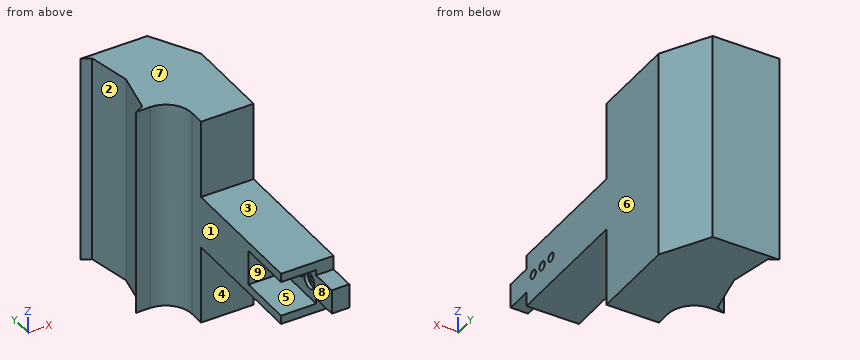
Autodesk Inventor part; units mm, degrees
ref_plane "Work Plane1" through (0, 0, -15) normal (0, 0, 1) x (1, 0, 0)
ref_plane "YZ Plane" through (0, 0, 0) normal (1, 0, 0) x (0, 1, 0)
ref_plane "XZ Plane" through (0, 0, 0) normal (0, 1, 0) x (-1, 0, 0)
sketch "Sketch1" plane through (0, 0, 0) normal (0, 0, 1) x (1, 0, 0)
  line L0 (0, 0) -> (25, 0)
  line L1 (25, 0) -> (25, 40)
  line L2 (25, 40) -> (0, 40)
  line L3 (0, 40) -> (0, 0)
  dimension "d1" = 25
  dimension "d2" = 40
  dimension "d3" = 25
extrude "Extrusion1" add sketch "Sketch1" against normal blind 30
sketch "Sketch2" plane through (25, 0, 0) normal (1, 0, 0) x (0, 0, -1)
  line L0 (0, 0) -> (30, 0)
  circle A0 centre (15, 6.56) radius 2.46
extrude "Extrusion2" cut sketch "Sketch2" against normal blind 30
sketch "Sketch3" plane through (0, 0, 0) normal (-1, 0, 0) x (0, 0, 1)
  line L0 (0, 0) -> (-30, 0)
  line L1 (-25.05, 0) -> (-4.95, 0)
  line L2 (-4.95, 0) -> (-4.95, 33.12)
  line L3 (-4.95, 33.12) -> (-25.05, 33.12)
  line L4 (-25.05, 33.12) -> (-25.05, 0)
  dimension "d11" = 20.1
extrude "Extrusion3" cut sketch "Sketch3" against normal blind 20
sketch "Sketch4" plane through (0, 0, 0) normal (0, -1, 0) x (1, 0, 0)
  line L0 (20, -4.95) -> (20, -25.05)
  line L1 (20, -15) -> (25, -15)
  line L2 (25, 0) -> (25, -30)
  line L3 (20, -8.025) -> (25, -8.025)
  line L4 (25, -8.025) -> (25, -21.975)
  line L5 (25, -21.975) -> (20, -21.975)
  line L6 (20, -21.975) -> (20, -8.025)
  line L7 (20, -8.025) -> (25, -21.975) construction
  line L8 (25, -8.025) -> (20, -21.975) construction
  line L9 (25, -12.54) -> (25, -17.46)
  point P0 (0, 0)
  point P1 (22.5, -15)
  dimension "d14" = 13.95
extrude "Extrusion4" add sketch "Sketch4" along normal blind 15
sketch "Sketch5" plane through (20, 0, 0) normal (-1, 0, 0) x (0, 0, 1)
  circle A0 centre (-15, 6.56) radius 2.46
  circle A1 centre (-15, 6.56) radius 4.7025
  circle A2 centre (-15, 6.56) radius 2.46
  circle A3 centre (-15, 6.56) radius 2.46
  point P0 (0, 0)
  dimension "d17" = 9.405
extrude "Extrusion5" cut sketch "Sketch5" against normal blind 2.1
sketch "Sketch6" plane through (25, 0, 0) normal (1, 0, 0) x (0, 0, -1)
  circle A0 centre (15, 6.56) radius 4.7025
  line L0 (15, 6.56) -> (15, 23.56)
  circle A1 centre (15, 23.56) radius 2.46
  point P0 (0, 0)
  dimension "d20" = 17
  dimension "d21" = 4.92
extrude "Extrusion6" cut sketch "Sketch6" against normal blind 10 contours A1
sketch "Sketch7" plane through (20, 0, 0) normal (-1, 0, 0) x (0, 0, 1)
  circle A0 centre (-15, 23.56) radius 2.46
  circle A1 centre (-15, 23.56) radius 4.7025
  point P0 (0, 0)
  dimension "d24" = 9.405
extrude "Extrusion7" cut sketch "Sketch7" against normal blind 2.1
sketch "Sketch9" plane through (25, 0, 0) normal (1, 0, 0) x (0, 0, -1)
  circle A0 centre (15, 6.56) radius 2.46
  circle A1 centre (15, 6.56) radius 2.46
  circle A2 centre (15, 23.56) radius 2.46
  circle A3 centre (15, 23.56) radius 2.46
  line L0 (30, 40) -> (30, 0)
  line L1 (30, 0) -> (30, 40)
  line L2 (30, 40) -> (0, 40)
  line L3 (0, 40) -> (0, 0)
  line L4 (0, 0) -> (8.025, 0)
  line L5 (21.975, 0) -> (21.975, -15)
  line L6 (21.975, -15) -> (8.025, -15)
  line L7 (8.025, -15) -> (8.025, 0)
  line L8 (0, 0) -> (8.025, 0)
  line L9 (21.975, 0) -> (30, 0)
extrude "Extrusion8" add sketch "Sketch9" along normal blind 5
sketch "Sketch10" plane through (0, 40, 0) normal (0, 1, 0) x (1, 0, 0)
  line L0 (0, 30) -> (30, 30)
  line L1 (30, 0) -> (0, 0)
  line L2 (0, 30) -> (30, 30)
  line L3 (30, 30) -> (30, 0)
  line L4 (30, 0) -> (0, 0)
  line L5 (0, 0) -> (0, 30)
extrude "Extrusion9" add sketch "Sketch10" along normal blind 30
sketch "Sketch12" plane through (30, 0, 0) normal (1, 0, 0) x (0, 0, -1)
  circle A0 centre (15, 6.56) radius 2.46
  line L0 (15, 6.56) -> (15, 15.06)
  circle A1 centre (15, 15.06) radius 2.525
  point P0 (0, 0)
  dimension "d31" = 8.5
  dimension "d33" = 5.05
extrude "Extrusion10" cut sketch "Sketch12" against normal blind 30 contours A1
sketch "Sketch14" plane through (0, 0, 0) normal (0, 0, 1) x (1, 0, 0)
  line L0 (30, 70) -> (0, 70)
  line L1 (0, 70) -> (0, 85)
  line L2 (-15, 100) -> (-23, 100)
  line L3 (30, 0) -> (30, 70)
  line L4 (30, 122.5) -> (30, 70)
  arc A0 (0, 85) -> (-15, 100) centre (-15, 85) ccw
  line L5 (30, 105) -> (30, 100)
  line L6 (-23, 153) -> (15, 153)
  line L7 (-18, 150.5) -> (-23, 153)
  line L8 (-18, 102.5) -> (-23, 100)
  line L9 (-18, 102.5) -> (-13, 126.5)
  line L10 (-13, 126.5) -> (-18, 150.5)
  line L11 (30, 126.5) -> (15, 153)
  line L12 (30, 122.5) -> (30, 126.5)
  point P0 (0, 0)
  point P1 (0, 100)
  dimension "d47" = 30
  dimension "d54" = 15
extrude "Extrusion12" add sketch "Sketch14" against normal blind 30
sketch "Sketch15" plane through (0, 0, -25.05) normal (-1, 0, 0) x (0, 0, 1)
  line L0 (0, 33.12) -> (20.1, 33.12)
  line L1 (20.1, 33.12) -> (20.1, 0)
  line L2 (0, 33.12) -> (20.1, 33.12)
  line L3 (20.1, 33.12) -> (20.1, 31.1)
  line L4 (20.1, 31.1) -> (0, 31.1)
  line L5 (0, 31.1) -> (0, 33.12)
  point P0 (25.05, 0)
  dimension "d57" = 2.02
extrude "Extrusion13" add sketch "Sketch15" against normal blind 20
sketch "Sketch25" plane through (0, 0, 0) normal (0, 0, 1) x (1, 0, 0)
  line L0 (-15, 100) -> (-23, 100)
  line L1 (-15, 100) -> (-23, 100)
  line L2 (-23, 100) -> (-18, 102.5)
  line L3 (-23, 100) -> (-18, 102.5)
  line L4 (-18, 102.5) -> (-13, 126.5)
  line L5 (-18, 102.5) -> (-13, 126.5)
  line L6 (-13, 126.5) -> (-18, 150.5)
  line L7 (-13, 126.5) -> (-18, 150.5)
  line L8 (-18, 150.5) -> (-23, 153)
  line L9 (-18, 150.5) -> (-23, 153)
  line L10 (-23, 153) -> (15, 153)
  line L11 (-23, 153) -> (15, 153)
  line L12 (15, 153) -> (30, 126.5)
  line L13 (15, 153) -> (30, 126.5)
  line L14 (30, 126.5) -> (30, 76.5)
  line L15 (30, 0) -> (30, 126.5)
  line L16 (30, 76.5) -> (0, 76.5)
  arc A0 (0, 85) -> (-15, 100) centre (-15, 85) ccw
  line L17 (0, 76.5) -> (0, 85)
  line L18 (0, 85) -> (0, 0)
  arc A1 (0, 85) -> (-15, 100) centre (-15, 85) ccw
  dimension "d90" = 50
extrude "Extrusion14" add sketch "Sketch25" along normal blind 45
ref_plane "Work Plane1" through (0, 0, -15) normal (0, 0, 1) x (1, 0, 0)
mirror "Mirror1" about plane through (0, 0, -15) normal (0, 0, 1) of "Extrusion14"
properties part number "rec_a_48mm_x_120mm"
Read the model definition and answer for the solid it produces. Units are mm, in the model's axes. Face numbers are marked on the shaded views. A direction names the side the tool comes from. Give positions to 0.01 mm unless a question says otherwise; leave off trailing zeros. Loops run counter-clockwise (first coordinate to the right, second up) from the corner with the lowest first, then second, coordinate; pieces in that order, holes last.
Item 1: Find the intervals of material crossed by line 1 along Z through (x, y) = (21, 23); line 2 along Z through (x, y) = (24.25, 23.56); line 3 along Y through (x, z) = (25.25, -15) (3 decimals), in increasing order.
Item 2: The part is cut by section A-A (z = -15). Give the number of separate pieces and of enclosed holes in the cut face, and give its area (3 significant figures).
Item 3: The part is cut by section D-D (z = -39.5). Write down the section's boundary in (x, y), and give its area (3 significant figures).
Item 4: The part is cut by section C-C (x = 12.5). Write down the section's boundary in (y, z).
Item 5: The mould has two halves that part along Z. Classify the marked faces 6, 7, 8 and 9: released by +Z, released by -Z, zero draft, split by the parting line, or undercut.
Item 6: The part is cut by section B-B (y = 15.06). Write down the section's boundary in (x, z) (3 decimals), and give its area (4 significant figures).
Item 7: For the marked faces 1, 2, 3, 4 and 5, determine the directions among +Z, -Z, +X, -X, +Y, -Y from which every point of the face is accessible in a straight line to the end or side of a thin tool.
Item 8: Each of these flat-tipped pins is pushed along its axis until it touches: pin 1 Ø24 at (x, z) = (19.5, -57.5) entering from -Y; pin 2 Ø10 at (x, z) = (7, -10.5) entering from -Y; pin 3 Ø5 at (x, y) = (11.5, 52) entering from -Z. Where does it stop, or does it pass through?
Taken from the geometry:
1. line 1: z = -30 to -19.67, -10.33 to 0
1. line 2: z = -30 to -17.46, -12.54 to 0
1. line 3: y = -15 to 4.1, 9.02 to 12.535, 17.585 to 21.1, 26.02 to 134.892
2. separate pieces: 4
2. enclosed holes: 0
2. area: 4,650 mm2
3. outline: (-23, 100) - (-15, 100) arc R15 cw to (0, 85) - (0, 76.5) - (30, 76.5) - (30, 126.5) - (15, 153) - (-23, 153) - (-18, 150.5) - (-13, 126.5) - (-18, 102.5) - close
3. area: 2,990 mm2
4. outline: (0, -30) - (76.5, -30) - (76.5, -75) - (153, -75) - (153, 45) - (76.5, 45) - (76.5, 0) - (0, 0) - (0, -4.95) - (31.1, -4.95) - (31.1, -25.05) - (0, -25.05) - close
5. face 6: zero draft
5. face 7: released by +Z
5. face 8: undercut
5. face 9: undercut
6. outline: (0, -30) - (30, -30) - (30, -17.525) - (20, -17.525) - (20, -25.05) - (0, -25.05) - close; (0, -4.95) - (20, -4.95) - (20, -12.475) - (30, -12.475) - (30, 0) - (0, 0) - close
6. area: 447.5 mm2
7. face 1: +Z, -Z, -X, -Y
7. face 2: +Z, -Z, -X
7. face 3: +Z, +X, -X, -Y
7. face 4: -Z, +X, -X, -Y
7. face 5: -X, -Y
8. pin 1: stops at y = 76.5
8. pin 2: stops at y = 31.1
8. pin 3: stops at z = -30
